The model under review builds one solid part; all positions refer to its coordinate system, in mm. A direction names the side the tool comes from. Give positions to 0.01 mm unless a question says otherwise; leave off trailing zeros. Order: outer loops, then holes, each group sorted by start corner. A loop starts at its lowest first (then second) coordinate and runs counter-clockwise, first axis right, second up. Notation, with made-up numbers: (-35, 3.5) - (-18, 3.5) arc R9 ccw to (-18, 7.5) - close; hole circle Ø1 at (39.5, 33). An arc over 180 degrees is marked (long way). Use CSV: the item, a comma, the result in double quotes. Start each with the question number.
1. Take a section at C-C, the plane x = -6.25. State the section outline as (y, z) points, then the cut area to 3 significant figures.
2. Take a section at A-A, the plane z = 0. State the section outline as (x, y) points, then the cut area to 3 significant figures.
3. For pin 1 (5 mm diameter, centred on y = 0, z = 0.5, fed in from +X); pin 2 (2 mm diameter, centred on x = -4.5, y = 4.5, fed in from -Z), all flat-tipped, find the tip position at first contact; note any pin that passes through.
4. Machinability: for faces 1 (the flat face through (0, -6.35, 0)), 2 (the flat face through (0.178, -1.233, 2.175)), which of the approach directions +Z, -Z, +X, -X, +Y, -Y give a long, thin tool a straight path to every point of the face, cutting with its end or side? Answer none if there is none.
5. Take a section at D-D, the plane z = -4.25. State the section outline as (x, y) points.
6. Take a section at B-B, the plane y = 2. State the section outline as (x, z) points, then the cut area to 3 significant figures.
7. Draft analysis for pull direction Z (two halves, no side actions). For faces 3 (the flat face through (12.7, 0.1, -3.2)), 4 (the flat face through (0.178, 1.233, -2.175)), 5 (the flat face through (0.178, 3.219, 5.474)), 6 (the flat face through (0, 2.5, 0)), state which applies: released by +Z, released by -Z, zero draft, split by the parting line, or undercut.
8. To check wall thickness, follow line 1 (Y direction, x = 5.25, z = 1); line 2 (Z direction, x = -11.5, y = -1) (3 decimals); line 3 (Z direction, x = 11, y = 1.75). State the ranges of each line that lie inside material, in increasing order. Write a range as [from, to].
```python
from build123d import *

# Parameters (mm, degrees)
BOSS_EXTRUDE1_DEPTH = 12.7


with BuildPart() as part:
    # Sketch1 → Boss-Extrude1 (new, symmetric)
    with BuildSketch(Plane(origin=(0, 0, 0), x_dir=(0, 0, -1), z_dir=(1, 0, 0))):
        Polygon((7.332348419, 0), (3.666174209, 6.35), (-3.666174209, 6.35), (-7.332348419, 0), (-3.666174209, -6.35), (3.666174209, -6.35), align=None)
        Polygon((2.886751346, 0), (1.443375673, 2.5), (-1.443375673, 2.5), (-2.886751346, 0), (-1.443375673, -2.5), (1.443375673, -2.5), align=None, mode=Mode.SUBTRACT)
    extrude(amount=BOSS_EXTRUDE1_DEPTH, both=True)


solid = part.part
```
Determined:
1,outline,"(-6.35, -3.67) - (0, -7.33) - (6.35, -3.67) - (6.35, 3.67) - (0, 7.33) - (-6.35, 3.67) - close; hole (-2.5, -1.44) - (0, -2.89) - (2.5, -1.44) - (2.5, 1.44) - (0, 2.89) - (-2.5, 1.44) - close"
1,area,"118 mm²"
2,outline,"(-12.7, -6.35) - (12.7, -6.35) - (12.7, -2.5) - (-12.7, -2.5) - close; (-12.7, 2.5) - (12.7, 2.5) - (12.7, 6.35) - (-12.7, 6.35) - close"
2,area,"196 mm²"
3,pin 1,"stops at x = 12.7"
3,pin 2,"stops at z = -5.31"
4,face 1,"+Z, -Z, +X, -X, -Y"
4,face 2,"+X, -X"
5,outline,"(-12.7, -5.34) - (12.7, -5.34) - (12.7, 5.34) - (-12.7, 5.34) - close"
6,outline,"(-12.7, -6.18) - (12.7, -6.18) - (12.7, -1.73) - (-12.7, -1.73) - close; (-12.7, 1.73) - (12.7, 1.73) - (12.7, 6.18) - (-12.7, 6.18) - close"
6,area,"226 mm²"
7,face 3,"zero draft"
7,face 4,"undercut"
7,face 5,"released by +Z"
7,face 6,"undercut"
8,line 1,"y = [-6.35, -2.5], [2.5, 6.35]"
8,line 2,"z = [-6.755, -2.309], [2.309, 6.755]"
8,line 3,"z = [-6.32, -1.88], [1.88, 6.32]"
